```python
from build123d import *

# Parameters (mm, degrees)
SKETCH_W        = 20
SKETCH_H        = 20
PAD_DEPTH       = 4.5
SKETCH001_R     = 1.7
POCKET_DEPTH    = 5
SKETCH002_R     = 2.8
POCKET001_DEPTH = 2.7
SKETCH003_W     = 4
SKETCH003_H     = 19.972413
PAD001_DEPTH    = 15


with BuildPart() as part:
    # Sketch → Pad (new body)
    with BuildSketch(Plane.XY):
        Rectangle(SKETCH_W, SKETCH_H)
    extrude(amount=PAD_DEPTH)

    # Sketch001 (on Face6 of Pad) → Pocket (cut)
    with BuildSketch(Plane.XY.offset(4.5)):
        Circle(SKETCH001_R)
    extrude(amount=-POCKET_DEPTH, mode=Mode.SUBTRACT)

    # Sketch002 (on Face5 of Pocket) → Pocket001 (cut)
    with BuildSketch(Plane.XY.offset(4.5)):
        Circle(SKETCH002_R)
    extrude(amount=-POCKET001_DEPTH, mode=Mode.SUBTRACT)

    # Sketch003 (on Face5 of Pocket001) → Pad001 (join)
    with BuildSketch(Plane.XY.offset(4.5)):
        with Locations((-8, 0.013794)):
            Rectangle(SKETCH003_W, SKETCH003_H)
    extrude(amount=PAD001_DEPTH)


solid = part.part
```
The listing builds one solid part. Answer for the finished solid, in the listing's coordinates (mm). A direction names the side the tool comes from. Give positions to 0.01 mm unless a question says otherwise; leave off trailing zeros. Order: outer loops, then holes, each group sorted by start corner. A loop starts at its lowest first (then second) coordinate and runs counter-clockwise, first axis right, second up. Notation, with made-up numbers: (54, 62) - (88, 62) arc R13 cw to (88, 84) - close; hole circle Ø5 at (-23, -40). An arc over 180 degrees is marked (long way). Answer in a Markdown table with one row per item. Add a question column.
Q1. For a pull along Y with two mould halves and no side action, classify faces 1 (the flat face through (0, -10, 2)), 2 (the flat face through (-8, 0, 19.5)), 3 (the flat face through (0, -2, 1.8)) as released by +Y, released by -Y, zero draft, split by the parting line, or undercut.
Q2. The part is cut by section B-B (z = 2.5). Determine the outline of the cut face in (x, y), then the cut area to 3 significant figures.
Q3. The part is cut by section D-D (x = 2.5). Determine the outline of the cut face in (y, z), then the cut area to 3 significant figures.
Q4. Which of the six approach directions +Z, -Z, +X, -X, +Y, -Y give full straight-line access (tool end or side, diameter ignored) to faces 4 (the flat face through (-6, 0, 12)), 5 (the flat face through (-8, -9.972, 12)), 6 (the cylindrical face through (-2.8, 0.1, 3.2)), 7 (the flat face through (-8, 10, 12))?
Q5. The part is cut by section C-C (y = 2.25). Determine the outline of the cut face in (x, z).
Q6. The part is cut by section A-A (x = 0). Determine the outline of the cut face in (y, z), then the cut area to 3 significant figures.
Q7. Find the intervals of material crossed by line 1 along Y through (x, z) = (0, 2.5); line 2 along Y through (x, z) = (0, 1.2); line 3 along Z through (x, y) = (8.5, -9), in increasing order. Write a range as [from, to].
Q8. Given P1, Ø4.5, axis at y = -4, z = 13, coming from the +X side; P2, Ø6, axis at x = -0.5, y = -1.5, coming from the +Z side; P3, Ø3, axis at x = -7, z = 15, coming from the -Y side; P4, Ø2, axis at x = 0, y = 0, coming from the -Z side, each flat-ended and moving along its own axis, determine where each tip first touches the part or whether it passes through.
Determined:
| question | item | result |
|---|---|---|
| 1 | face 1 | released by -Y |
| 1 | face 2 | zero draft |
| 1 | face 3 | undercut |
| 2 | outline | (-10, -10) - (10, -10) - (10, 10) - (-10, 10) - close; hole circle Ø5.6 at (0, 0) |
| 2 | area | 375 mm² |
| 3 | outline | (-10, 0) - (10, 0) - (10, 4.5) - (1.26, 4.5) - (1.26, 1.8) - (-1.26, 1.8) - (-1.26, 4.5) - (-10, 4.5) - close |
| 3 | area | 83.2 mm² |
| 4 | face 4 | +Z, +X, +Y, -Y |
| 4 | face 5 | +Z, +X, -X, -Y |
| 4 | face 6 | +Z |
| 4 | face 7 | +Z, -Z, +X, -X, +Y |
| 5 | outline | (-10, 0) - (10, 0) - (10, 4.5) - (1.67, 4.5) - (1.67, 1.8) - (-1.67, 1.8) - (-1.67, 4.5) - (-6, 4.5) - (-6, 19.5) - (-10, 19.5) - close |
| 6 | outline | (-10, 0) - (-1.7, 0) - (-1.7, 1.8) - (-2.8, 1.8) - (-2.8, 4.5) - (-10, 4.5) - close; (1.7, 0) - (10, 0) - (10, 4.5) - (2.8, 4.5) - (2.8, 1.8) - (1.7, 1.8) - close |
| 6 | area | 68.8 mm² |
| 7 | line 1 | y = [-10, -2.8], [2.8, 10] |
| 7 | line 2 | y = [-10, -1.7], [1.7, 10] |
| 7 | line 3 | z = [0, 4.5] |
| 8 | P1 | stops at x = -6 |
| 8 | P2 | stops at z = 4.5 |
| 8 | P3 | stops at y = -9.97 |
| 8 | P4 | passes through |
